Model file for the job. Use its own axes, mm. Face numbers are marked on the shaded views. A direction names the side the tool comes from. Coordinates: 2 decimals unless noted, no trailing zeros. Write each loop counter-clockwise with the first axis right and the second up, starting at its lowest first coordinate (ties: lowest second). Pieces come first, ordered by that corner, then holes.
Q1. Band-saw the part on A-A, the plane x = 2.5. Write the cut outline in (y, z).
Q2. Band-saw the part on D-D, the plane x = -12.5. Write the cut outline in (y, z).
Q3. Which spindle directions (+Z, -Z, +X, -X, +Y, -Y) get a long thin tool onto all of the face, cutting with end or side? Do the marked faces 1, 2 and 3. Say none if no direction does.
Q4. Pin check, flat tips, straight feed: P1, Ø0.6, axis at x = 12.5, z = 0.5, coming from the +Y side; P2, Ø4, axis at y = -3.5, z = 9.5, coming from the -X side; P3, Ø2, axis at y = 12.5, z = 1.5, coming from the +X side. Stop position of each tip, or through.
Q5. Drill centre lines: probe 1 along Z at (x, y) = (-1, -1.75); probe 2 along Z at (x, y) = (4.5, -12.25); probe 3 along X at (y, z) = (-6, 10.5). Where is each one in solid material? Low to high.
Q6. Pull direction Z, two halves, no side cores. Call the marked faces 4, 5 and 6: released by +Z, released by -Z, zero draft, split by the parting line, or undercut.
Q7. Band-saw the part on B-B, the plane y = 0.5. Write the cut outline in (x, z), plus the area to 4 significant figures.
Q8. Band-saw the part on C-C, the plane z = 7.75. Write the cut outline in (x, y), plus the area to 3 significant figures.
from build123d import *

# Parameters (mm, degrees)
SKETCH1_W           = 29
SKETCH1_H           = 29
BOSS_EXTRUDE1_DEPTH = 20
SKETCH2_W           = 26
SKETCH2_H           = 16
CUT_EXTRUDE1_DEPTH  = 26
CUT_EXTRUDE2_DEPTH  = 21
SKETCH4_W           = 10
SKETCH4_H           = 6
CUT_EXTRUDE3_DEPTH  = 30
SKETCH5_W           = 6
SKETCH5_H           = 10
CUT_EXTRUDE4_DEPTH  = 30


with BuildPart() as part:
    # Sketch1 → Boss-Extrude1 (new body)
    with BuildSketch(Plane.XY):
        Rectangle(SKETCH1_W, SKETCH1_H)
    extrude(amount=BOSS_EXTRUDE1_DEPTH)

    # Sketch2 → Cut-Extrude1 (cut)
    with BuildSketch(Plane(origin=(0, 14.5, 0), x_dir=(1, 0, 0), z_dir=(0, 1, 0))):
        with Locations((1.5, -10)):
            Rectangle(SKETCH2_W, SKETCH2_H)
    extrude(amount=-CUT_EXTRUDE1_DEPTH, mode=Mode.SUBTRACT)

    # Sketch3 → Cut-Extrude2 (cut, through all)
    with BuildSketch(Plane.XY.offset(20)):
        Polygon((-7.5, 14.5), (-7.5, 11), (11, -7.5), (14.5, -7.5), (14.5, 14.5), align=None)
    extrude(amount=-CUT_EXTRUDE2_DEPTH, mode=Mode.SUBTRACT)

    # Sketch4 → Cut-Extrude3 (cut, through all)
    with BuildSketch(Plane.XZ.offset(14.5)):
        with Locations((0.5, 10)):
            Rectangle(SKETCH4_W, SKETCH4_H)
    extrude(amount=-CUT_EXTRUDE3_DEPTH, mode=Mode.SUBTRACT)

    # Sketch5 → Cut-Extrude4 (cut, through all)
    with BuildSketch(Plane.ZY.offset(14.5)):
        with Locations((10, 0.5)):
            Rectangle(SKETCH5_W, SKETCH5_H)
    extrude(amount=-CUT_EXTRUDE4_DEPTH, mode=Mode.SUBTRACT)


solid = part.part
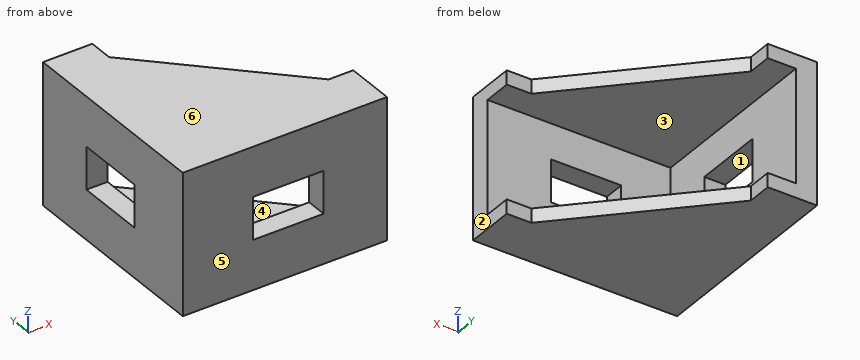
Answer sheet:
1. outline: (-14.5, 0) - (1, 0) - (1, 2) - (-11.5, 2) - (-11.5, 7) - (-14.5, 7) - close; (-14.5, 13) - (-11.5, 13) - (-11.5, 18) - (1, 18) - (1, 20) - (-14.5, 20) - close
2. outline: (-14.5, 0) - (14.5, 0) - (14.5, 20) - (-14.5, 20) - close; hole (-4.5, 7) - (5.5, 7) - (5.5, 13) - (-4.5, 13) - close
3. face 1: +X, -X
3. face 2: +Z, -Z, +X, +Y, -Y
3. face 3: +X, +Y
4. P1: stops at y = -7.5
4. P2: stops at x = -14.5
4. P3: stops at x = -7.5
5. probe 1: z = 0 to 2, 18 to 20
5. probe 2: z = 0 to 7, 13 to 20
5. probe 3: x = -14.5 to -11.5
6. face 4: undercut
6. face 5: zero draft
6. face 6: released by +Z
7. outline: (-14.5, 0) - (3, 0) - (3, 2) - (-11.5, 2) - (-11.5, 7) - (-14.5, 7) - close; (-14.5, 13) - (-11.5, 13) - (-11.5, 18) - (3, 18) - (3, 20) - (-14.5, 20) - close
7. area: 100.0 mm2
8. outline: (-14.5, -14.5) - (-4.5, -14.5) - (-4.5, -11.5) - (-11.5, -11.5) - (-11.5, -4.5) - (-14.5, -4.5) - close; (-14.5, 5.5) - (-11.5, 5.5) - (-11.5, 14.5) - (-14.5, 14.5) - close; (5.5, -14.5) - (14.5, -14.5) - (14.5, -11.5) - (5.5, -11.5) - close
8. area: 105 mm2
